Read the model definition and answer for the solid it produces. Units are mm, in the model's axes. Face numbers are marked on the shaded views. A direction names the side the tool comes from. Round coordinates to 2 decimals unless told otherwise and drop trailing zeros. Write each loop counter-clockwise with the first axis right and the second up, starting at its lowest first coordinate (ties: lowest second). Pieces come first, ordered by that corner, then holes. Notation, with made-up numbers: (-21.5, -36) -> (26.5, -36) arc R23 cw to (26.5, -7) -> close; hole circle Ø11 at (-11.5, 43). An arc over 180 degrees is marked (long way). Return JSON: item names as keys, results as strings.
from build123d import *

# Parameters (mm, degrees)
SKETCH1_R           = 1.5
BOSS_EXTRUDE1_DEPTH = 13.75
SKETCH2_R           = 2.25
BOSS_EXTRUDE2_DEPTH = 11.5
BOSS_EXTRUDE3_START = 2.75
SKETCH3_R           = 1.5
BOSS_EXTRUDE3_DEPTH = 2.75


with BuildPart() as part:
    # Sketch1 → Boss-Extrude1 (new body)
    with BuildSketch(Plane(origin=(0, 0, 0), x_dir=(1, 0, 0), z_dir=(0, 1, 0))):
        with Locations(Location((0, 0, 0), (0, 0, 270))):
            Circle(SKETCH1_R)
    extrude(amount=-BOSS_EXTRUDE1_DEPTH)

    # Sketch2 → Boss-Extrude2 (add)
    with BuildSketch(Plane(origin=(0, 0, 0), x_dir=(1, 0, 0), z_dir=(0, 1, 0))):
        with Locations(Location((0, 0, 0), (0, 0, 270))):
            Circle(SKETCH2_R)
    extrude(amount=BOSS_EXTRUDE2_DEPTH)

    # Sketch3 → Boss-Extrude3 (add)
    with BuildSketch(Plane(origin=(0, 11.5, 0), x_dir=(1, 0, 0), z_dir=(0, 1, 0)).offset(BOSS_EXTRUDE3_START)):
        with Locations(Location((0, 0, 0), (0, 0, 270))):
            Circle(SKETCH3_R)
    extrude(amount=-BOSS_EXTRUDE3_DEPTH)


solid = part.part
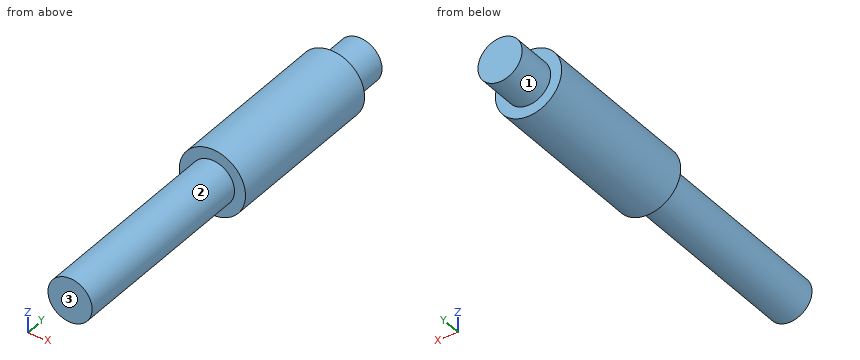
Item 1: A tool of negligible diameter and unlimited length cuts with its end or side. For the marked faces 1, 2 and 3, from which of +Z, -Z, +X, -X, +Y, -Y can it reach the whole face along a straight path? Write none if from no direction.
Worked answers:
{"face 1": "+Y", "face 2": "-Y", "face 3": "+Z, -Z, +X, -X, -Y"}
Item 2: Section C-C (y = -9.5) is taken. Give the vertices of the cut face in (x, z).
Worked answers:
{"outline": "circle Ø3 at (0, 0)"}
Item 3: Section B-B (x = 0) is taken. Give the vertices of the cut face in (y, z), then the cut area to 3 significant figures.
Worked answers:
{"outline": "(-13.75, -1.5) -> (0, -1.5) -> (0, -2.25) -> (11.5, -2.25) -> (11.5, -1.5) -> (14.25, -1.5) -> (14.25, 1.5) -> (11.5, 1.5) -> (11.5, 2.25) -> (0, 2.25) -> (0, 1.5) -> (-13.75, 1.5) -> close", "area": "101 mm2"}
Item 4: A flat-ended cylindrical pin translates along its axis: pin 1 (1.5 mm diameter, centred on y = -6, z = -0.5, fed in from +X). Find the tip coordinate at first contact, or state that the pin passes through.
Worked answers:
{"pin 1": "stops at x = 1.5"}
Item 5: Section A-A (z = 0) is taken. Give the vertices of the cut face in (x, y).
Worked answers:
{"outline": "(-2.25, 0) -> (-1.5, 0) -> (-1.5, -13.75) -> (1.5, -13.75) -> (1.5, 0) -> (2.25, 0) -> (2.25, 11.5) -> (1.5, 11.5) -> (1.5, 14.25) -> (-1.5, 14.25) -> (-1.5, 11.5) -> (-2.25, 11.5) -> close"}
Item 6: Section D-D (x = -1.8) is taken. Give the vertices of the cut face in (y, z).
Worked answers:
{"outline": "(0, -1.35) -> (11.5, -1.35) -> (11.5, 1.35) -> (0, 1.35) -> close"}
Item 7: Straight lines are drawn through the part: L1, parallel to Y at x = 2.05, z = 0; L2, parallel to X at y = 4, z = 1.9; L3, parallel to X at y = 9.75, z = -0.35. For each, find the intervals that lie inside material, in ascending order. Write a range as [from, to].
Worked answers:
{"L1": "y = [0, 11.5]", "L2": "x = [-1.21, 1.21]", "L3": "x = [-2.22, 2.22]"}
